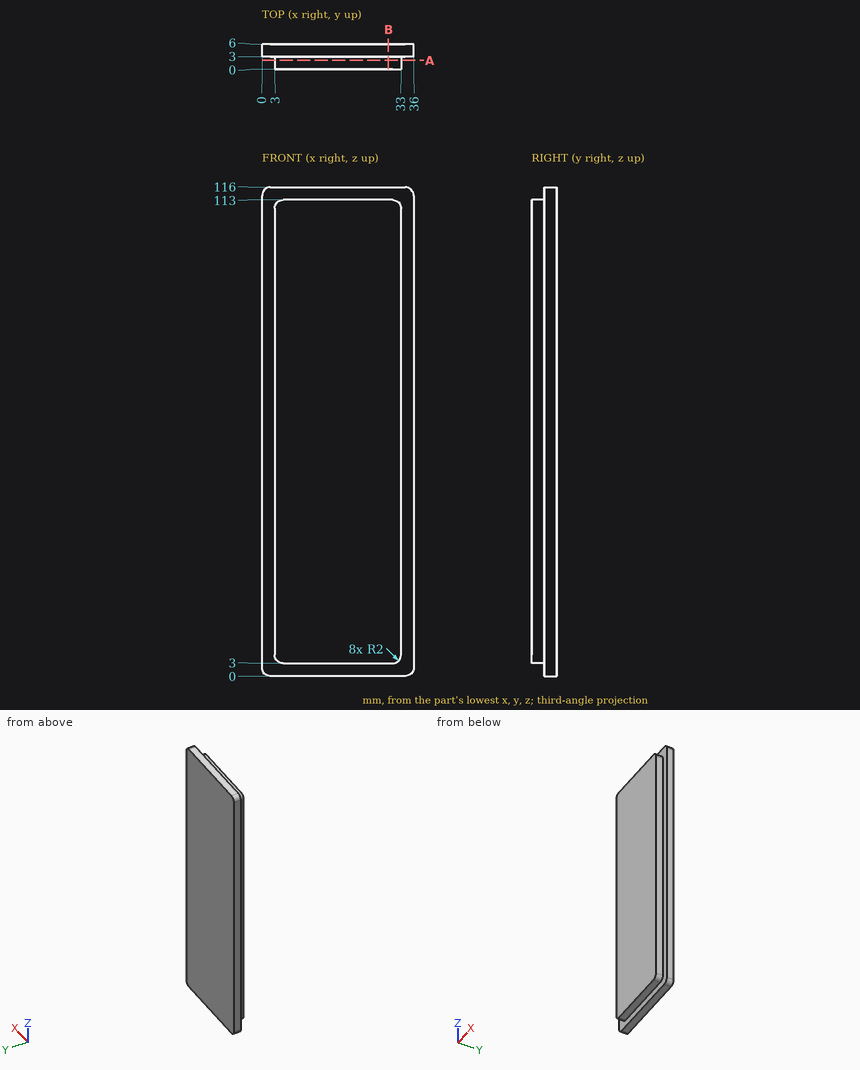
Source: three-view drawing plus pictorial views. Frame: mm from the lowest corner of the part. Coordinates: 2 decimals unless noted, no trailing zeros. Loops run counter-clockwise (first coordinate to the right, second up) from the corner with the lowest first, then second, coordinate; pieces in that order, holes last. Notation, with made-up numbers: (27.25, 33.5) -> (70.25, 33.5) arc R29 ccw to (70.25, 57.5) -> close; hole circle Ø3 at (-11, -8). An arc over 180 degrees is marked (long way). Write each question's results on one line, items separated by ' | '. Start each with the question number.
Q1. Ray query, line 1 (X direction, y = 2.8, z = 69); line 2 (Z direction, x = 22.5, y = 0.8); line 3 (Z direction, x = 35.5, y = 4.35). Return the intervals inside material, ascending. Write a range as from..to.
Q2. Section B-B, the plane x = 30. Return the cut outline in (y, z), plus the area to 3 significant figures.
Q3. Section A-A, the plane y = 2.1. Return the cut outline in (x, z).
Q4. Pin query (flat end, axial travel): pin 1 (1.5 mm diameter, centred on y = 1, z = 69, fed in from +X); pin 2 (1.5 mm diameter, centred on y = 1.5, z = 59, fed in from -X); pin 3 (3.5 mm diameter, centred on x = 12, y = 1, fed in from -Z). Return the tip coordinate at first contact, or that it passes through.
Found:
1) line 1: 3..33 | line 2: 3..113 | line 3: 0.68..115.32
2) outline: (0, 3) -> (3, 3) -> (3, 0) -> (6, 0) -> (6, 116) -> (3, 116) -> (3, 113) -> (0, 113) -> close | area: 678 mm2
3) outline: (3, 5) arc R2 ccw to (5, 3) -> (31, 3) arc R2 ccw to (33, 5) -> (33, 111) arc R2 ccw to (31, 113) -> (5, 113) arc R2 ccw to (3, 111) -> close
4) pin 1: x = 33 | pin 2: x = 3 | pin 3: z = 3
